Can you work these out from the drawing? Everything is in mm from the part's minimum corner. Coordinates: 2 decimals unless noted, no trailing zeros. Write each loop counter-clockwise with the first axis right and the second up, starting at its lowest first coordinate (ties: lowest second). Pieces come first, ordered by that corner, then holes. Notation, with made-up numbers: M 8.25,-21 L 30.25,-21 A20 cw 30.25,-14 Z; hole C 35,-18 d11. An arc over 180 degrees is marked long. Use one line per item in the form item = value. Start each with the question number.
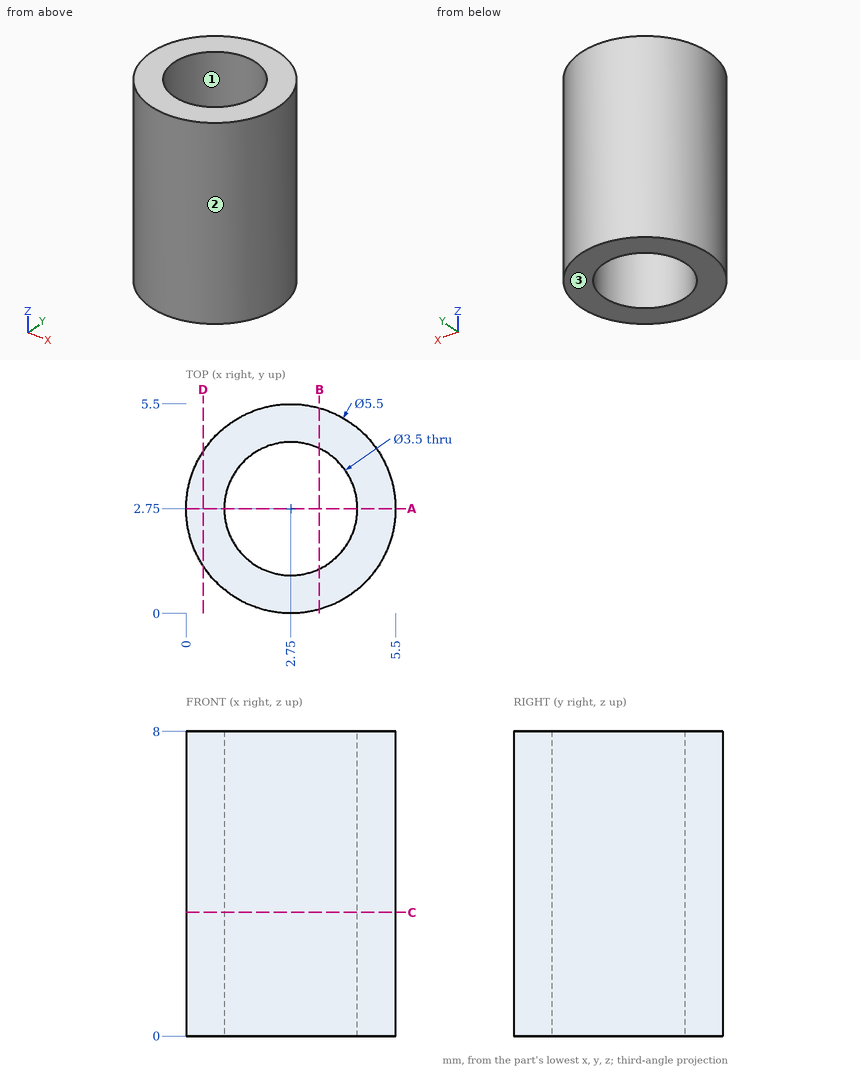
1) Please list where these lines run through material, in increasing order: line 1 (Y direction, x = 2.75, z = 3.75); line 2 (Y direction, x = 1.2, z = 1).
2) If we mould it in two halves opening along Y, with no side actions, what happens to the marked faces 1, 2 and 3? For each: +Y half, -Y half, draft (parallel to the pull), parting line (faces both ways), or undercut.
3) Suppose I cut it at B-B on x = 3.5. Please give me the cut outline in (y, z).
4) Suppose I cut it at A-A on y = 2.75. Please give me the cut outline in (x, z).
5) Suppose I cut it at C-C on z = 3.25. Please give me the cut outline in (x, y), and give its area (3 significant figures).
6) Will these pins go through, and if not, where does the flat tip stop? pin 1 Ø2 at (x, y) = (5, 1.5) entering from -Z; pin 2 Ø1.5 at (y, z) = (1.5, 4) entering from -X; pin 3 Ø1 at (y, z) = (1, 2.5) entering from +X.
7) Suppose I cut it at D-D on x = 0.45. Please give me the cut outline in (y, z).
Computed values:
q1.line_1 = 0 to 1, 4.5 to 5.5
q1.line_2 = 0.48 to 1.94, 3.56 to 5.02
q2.face_1 = undercut
q2.face_2 = parting line
q2.face_3 = draft
q3.outline = M 0.1,0 L 1.17,0 L 1.17,8 L 0.1,8 Z; M 4.33,0 L 5.4,0 L 5.4,8 L 4.33,8 Z
q4.outline = M 0,0 L 1,0 L 1,8 L 0,8 Z; M 4.5,0 L 5.5,0 L 5.5,8 L 4.5,8 Z
q5.outline = C 2.75,2.75 d5.5; hole C 2.75,2.75 d3.5
q5.area = 14.1 mm²
q6.pin_1 = 0
q6.pin_2 = 0.05
q6.pin_3 = 5.2
q7.outline = M 1.24,0 L 4.26,0 L 4.26,8 L 1.24,8 Z
